For this review, use the dimensioned drawing (mm, ordinates from the lowest corner) and the shaded views. Coordinates: 2 decimals unless noted, no trailing zeros. Order: outer loops, then holes, each group sorted by start corner. A loop starts at its lowest first (then second) coordinate and runs counter-clockwise, first axis right, second up. Notation, with made-up numbers: M 64.25,61.25 L 102.25,61.25 A22 cw 102.25,67.25 Z; hole C 45,26.25 d6. An arc over 180 degrees is marked long. Use one line per item in the form item = value. Start each with the question number.
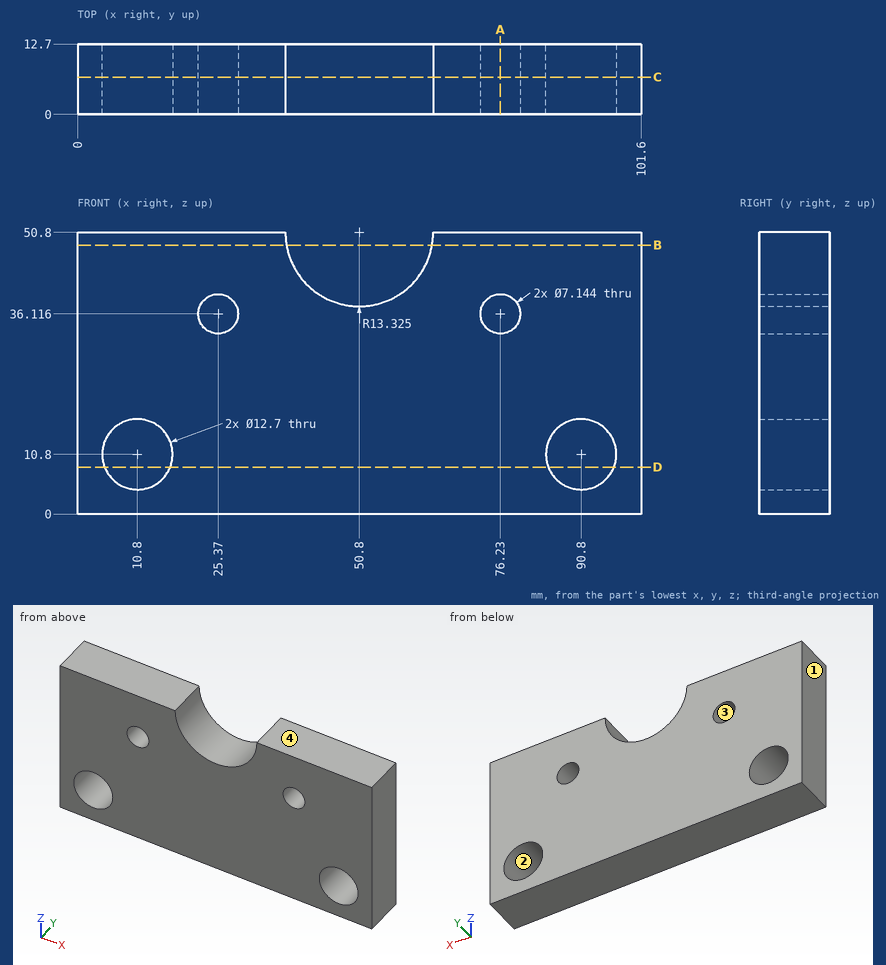
1. Consider section D-D, the plane z = 8.5. Write out the cut boundary in (x, y).
2. The part is to be moulded in two halves that separate along Z. For the marked faces 1, 2, 3 and 4, say which applies: pulls with the +Z half, pulls with the -Z half, needs draft (parallel to the pull), parting line crosses it, or undercut.
3. Consider section B-B, the plane z = 48.5. Write out the cut boundary in (x, y) (1 decimal).
4. Consider section A-A, the plane x = 76.23. Write out the cut boundary in (y, z).
5. To check wall thickness, follow line 1 (Z direction, x = 90.8, y = 6); line 2 (X direction, y = 7.75, z = 10); line 3 (X direction, y = 9.5, z = 39) (1 decimal). State the ranges of each line that lie inside material, in increasing order.
6. Consider section C-C, the plane y = 6.75. Give the number of separate pieces and of enclosed holes in the cut face, plus the area to 3 significant figures.
Answers follow:
q1.outline = M 0,0 L 4.88,0 L 4.88,12.7 L 0,12.7 Z; M 16.72,0 L 84.88,0 L 84.88,12.7 L 16.72,12.7 Z; M 96.72,0 L 101.6,0 L 101.6,12.7 L 96.72,12.7 Z
q2.face_1 = needs draft
q2.face_2 = undercut
q2.face_3 = undercut
q2.face_4 = pulls with the +Z half
q3.outline = M 0,0 L 37.7,0 L 37.7,12.7 L 0,12.7 Z; M 63.9,0 L 101.6,0 L 101.6,12.7 L 63.9,12.7 Z
q4.outline = M 0,0 L 12.7,0 L 12.7,32.54 L 0,32.54 Z; M 0,39.69 L 12.7,39.69 L 12.7,50.8 L 0,50.8 Z
q5.line_1 = 0 to 4.45, 17.15 to 50.8
q5.line_2 = 0 to 4.5, 17.1 to 84.5, 97.1 to 101.6
q5.line_3 = 0 to 23.3, 27.5 to 44.6, 57 to 74.1, 78.3 to 101.6
q6.separate_pieces = 1
q6.enclosed_holes = 4
q6.area = 4,550 mm²
